```python
from build123d import *

# Parameters (mm, degrees)
F1_DEPTH = 8.636
F3_D     = 3.556
F5_DEPTH = 25.4


with BuildPart() as f1:
    # F0 (on Front) → F1 (new body)
    with BuildSketch(Plane.XZ):
        with BuildLine():
            Line((-39.490599, 56.54397), (-42.455846, 60.334262))
            ThreePointArc((-42.455846, 60.334262), (-42.595136, 60.320247), (-42.671131, 60.202675))
            ThreePointArc((-42.671131, 60.202675), (-45.433619, 53.07891), (-49.732476, 46.762329))
            Line((-49.732476, 46.762329), (-45.894753, 47.265854))
            ThreePointArc((-45.894753, 47.265854), (-44.359586, 46.782597), (-43.033395, 45.870733))
            Line((-43.033395, 45.870733), (-40.480834, 43.487869))
            Line((-40.480834, 43.487869), (-36.865097, 42.211726))
            Line((-36.865097, 42.211726), (-35.26992, 40.350687))
            Line((-35.26992, 40.350687), (-35.26992, 36.170255))
            Line((-35.26992, 36.170255), (-37.580833, 35.163075))
            Line((-37.580833, 35.163075), (-46.559945, 36.170255))
            Line((-46.559945, 36.170255), (-52.048847, 37.195779))
            Line((-52.048847, 37.195779), (-53.439979, 34.539986))
            Line((-53.439979, 34.539986), (-51.661003, 18.294973))
            Line((-51.661003, 18.294973), (-51.661003, 14.98081))
            Line((-51.661003, 14.98081), (-52.724455, 10.638124))
            Line((-52.724455, 10.638124), (-51.022932, 7.44777))
            Line((-51.022932, 7.44777), (-49.108718, 5.746248))
            Line((-49.108718, 5.746248), (-47.003191, 6.949406))
            Line((-47.003191, 6.949406), (-44.897664, 9.054932))
            Line((-44.897664, 9.054932), (-44.897664, 11.010064))
            Line((-44.897664, 11.010064), (-46.401612, 14.98081))
            Line((-46.401612, 14.98081), (-47.602195, 18.323077))
            Line((-47.602195, 18.323077), (-45.334391, 29.303517))
            Line((-45.334391, 29.303517), (-37.631679, 27.457869))
            Line((-37.631679, 27.457869), (-29.565466, 8.868489))
            Line((-29.565466, 8.868489), (-41.40104, -6.316776))
            Line((-41.40104, -6.316776), (-40.112628, -9.657612))
            Line((-40.112628, -9.657612), (-20.918895, -25.618885))
            Line((-20.918895, -25.618885), (-19.961456, -27.996508))
            Line((-19.961456, -27.996508), (-20.918895, -31.849388))
            Line((-20.918895, -31.849388), (-20.392513, -35.308465))
            Line((-20.392513, -35.308465), (-18.362185, -33.456158))
            Line((-18.362185, -33.456158), (-17.008632, -32.150175))
            Line((-17.008632, -32.150175), (-10.893537, -24.137914))
            ThreePointArc((-10.893537, -24.137914), (-13.35981, -21.972545), (-16.342713, -20.603744))
            ThreePointArc((-16.342713, -20.603744), (-24.815375, -15.496005), (-30.766526, -7.592917))
            Line((-30.766526, -7.592917), (-21.195464, 3.466977))
            Line((-21.195464, 3.466977), (-6.674734, -0.787208))
            Line((-6.674734, -0.787208), (-15.962735, -9.781499))
            Line((-15.962735, -9.781499), (-15.962735, -11.829657))
            Line((-15.962735, -11.829657), (-6.730688, -19.544106))
            Line((-6.730688, -19.544106), (-4.248045, -18.667899))
            Line((-4.248045, -18.667899), (-7.509657, -11.641931))
            Line((-7.509657, -11.641931), (3.868554, -1.177071))
            Line((3.868554, -1.177071), (5.38615, 0.846392))
            Line((5.38615, 0.846392), (5.38615, 1.921356))
            Line((5.38615, 1.921356), (4.464583, 2.667227))
            Line((4.464583, 2.667227), (-10.695753, 9.356373))
            Line((-10.695753, 9.356373), (-11.397142, 11.017655))
            Line((-11.397142, 11.017655), (-10.18736, 13.336552))
            Line((-10.18736, 13.336552), (-8.770354, 13.934808))
            Line((-8.770354, 13.934808), (-8.770354, 16.013902))
            Line((-8.770354, 16.013902), (-10.18736, 17.962622))
            Line((-10.18736, 17.962622), (-18.269591, 38.380887))
            Line((-18.269591, 38.380887), (-14.161164, 43.704748))
            Line((-14.161164, 43.704748), (-4.64041, 24.543248))
            Line((-4.64041, 24.543248), (-3.257924, 23.054415))
            Line((-3.257924, 23.054415), (-1.556402, 23.054415))
            Line((-1.556402, 23.054415), (0.89488, 23.054415))
            Line((0.89488, 23.054415), (2.474027, 24.543248))
            Line((2.474027, 24.543248), (3.000409, 25.854964))
            Line((3.000409, 25.854964), (2.173235, 27.058123))
            Line((2.173235, 27.058123), (0.486221, 27.465567))
            Line((0.486221, 27.465567), (-0.942529, 27.058123))
            Line((-0.942529, 27.058123), (-2.728466, 27.058123))
            Line((-2.728466, 27.058123), (-5.468886, 39.159644))
            Line((-5.468886, 39.159644), (-9.891379, 49.272485))
            Line((-9.891379, 49.272485), (-12.826882, 53.211112))
            Line((-12.826882, 53.211112), (-13.20135, 53.563222))
            Line((-13.20135, 53.563222), (-13.536695, 53.563222))
            Line((-13.536695, 53.563222), (-13.782615, 53.501744))
            Line((-13.782615, 53.501744), (-13.911596, 53.357568))
            Line((-13.911596, 53.357568), (-15.284945, 52.576538))
            Line((-15.284945, 52.576538), (-17.14508, 51.778425))
            Line((-17.14508, 51.778425), (-19.250607, 49.296912))
            Line((-19.250607, 49.296912), (-22.991639, 46.002153))
            Line((-22.991639, 46.002153), (-25.414456, 44.81658))
            Line((-25.414456, 44.81658), (-26.532697, 43.852221))
            Line((-26.532697, 43.852221), (-28.234769, 42.931135))
            Line((-28.234769, 42.931135), (-29.056527, 43.291926))
            Line((-29.056527, 43.291926), (-30.184661, 45.565556))
            Line((-30.184661, 45.565556), (-28.773969, 46.265516))
            Line((-28.773969, 46.265516), (-28.800942, 46.998821))
            Line((-28.800942, 46.998821), (-30.88334, 50.958432))
            ThreePointArc((-30.88334, 50.958432), (-30.692044, 51.200237), (-30.552286, 51.475067))
            ThreePointArc((-30.552286, 51.475067), (-30.469588, 51.772006), (-30.447163, 52.079428))
            Line((-30.447163, 52.079428), (-30.995147, 51.97043))
            ThreePointArc((-30.995147, 51.97043), (-32.513604, 52.028513), (-33.906634, 52.635599))
            Line((-33.906634, 52.635599), (-35.530325, 53.740148))
            Line((-35.530325, 53.740148), (-33.031618, 57.413258))
            ThreePointArc((-33.031618, 57.413258), (-33.016248, 57.657381), (-33.222877, 57.788287))
            ThreePointArc((-33.222877, 57.788287), (-36.255309, 57.358332), (-39.185994, 56.468622))
            ThreePointArc((-39.185994, 56.468622), (-39.351294, 56.453752), (-39.490599, 56.54397))
        make_face()
    extrude(amount=F1_DEPTH)

    # F3 (through all)
    with Locations(Plane.XZ.offset(8.636)):
        with Locations((-14.032521, 49.561661)):
            Hole(F3_D / 2)

    # F4 (on face) → F5 (cut)
    with BuildSketch(Plane.XZ.offset(8.636)):
        Polygon((-36.247086, 50.90744), (-34.366347, 50.90744), (-33.865116, 52.420092), (-35.530989, 52.308187), align=None)
    extrude(amount=-F5_DEPTH, mode=Mode.SUBTRACT)


solid = f1.part
```
Could you check a few things on this model? Use its own coordinates, in mm. A direction names the side the tool comes from. Coordinates: 2 decimals unless noted, no trailing zeros. Write each loop counter-clockwise with the first axis right and the second up, starting at its lowest first coordinate (ties: lowest second). Pieces come first, ordered by that corner, then holes. Notation, with made-up numbers: (66, -12.5) - (113, -12.5) arc R15 cw to (113, 12.5) - close; hole circle Ø2 at (-6, -24). An arc over 180 degrees is marked (long way). Use a Markdown table: item, result.
Q1. Imagine slicing it at B-B (y = -2.75). Count the separate pieces of the cut face and the enclosed holes in it, and give its area (3 significant figures).
Geometry check:
| item | result |
|---|---|
| separate pieces | 1 |
| enclosed holes | 2 |
| area | 2,140 mm2 |
Q2. Which directions (+Z, -Z, +X, -X, +Y, -Y) give clear straight access to the entire face, cutting with the end or side of a thin tool? Please do faces 1 (the flat face through (-46.484, -4.258, 23.736)), 2 (the flat face through (-51.661, -4, 17)), 3 (the flat face through (4.6, -4.3, -0.2)).
Geometry check:
| item | result |
|---|---|
| face 1 | +Y, -Y |
| face 2 | -X, +Y, -Y |
| face 3 | -Z, +X, +Y, -Y |
Q3. Imagine slicing it at A-A (z = -4). List the corners of the cut face in (x, y) for me.
Geometry check:
| item | result |
|---|---|
| outline | (-39.6, -8.64) - (-27.66, -8.64) - (-27.66, 0) - (-39.6, 0) - close; (-9.99, -8.64) - (0.8, -8.64) - (0.8, 0) - (-9.99, 0) - close |
Q4. Thinking about a two-plate mould opening in Z: for faces 4 (the flat face through (-18.18, -4.26, 50.56)), 5 (the flat face through (-35.4, -4.26, 1.38)), 6 (the flat face through (-19.392, -4.258, -34.395)), which applies, +Z half, -Z half, draft (parallel to the pull), parting line (faces both ways), or undercut?
Geometry check:
| item | result |
|---|---|
| face 4 | +Z half |
| face 5 | undercut |
| face 6 | -Z half |
Q5. I'm going to push flat-ended pins straight in: pin 1 Ø3.5 at (y, z) = (-4.5, 17) entering from -X; pin 2 Ø4 at (y, z) = (-5.5, 4) entering from -X; pin 3 Ø3 at (x, y) = (-30, -3.5) entering from -Z; pin 4 Ø8 at (x, z) = (-39, 9) entering from +Y. Where does each tip first touch, or does it pass through?
Geometry check:
| item | result |
|---|---|
| pin 1 | stops at x = -51.71 |
| pin 2 | stops at x = -49.39 |
| pin 3 | stops at z = -19.31 |
| pin 4 | passes through |
Q6. Please list where these lines run through material, in increasing order: L1, parallel to Z at x = -8, y = -4.25; L2, parallel to Z at x = -9.5, y = -7.25; L3, parallel to Z at x = -37, y = -5.25.
Geometry check:
| item | result |
|---|---|
| L1 | z = -18.48 to -2.07, -0.4 to 8.17, 31.3 to 44.95 |
| L2 | z = -17.23 to -3.52, 0.04 to 8.83, 13.63 to 17.02, 34.32 to 48.38 |
| L3 | z = -12.25 to -0.67, 26 to 35.42, 42.26 to 57.18 |
